Check sheet for the modelled part. Datum: model origin and axes. Units: mm. Face numbers are marked on the shaded views. A direction names the side the tool comes from. Give positions to 0.01 mm unless a question says otherwise; leave off trailing zeros. Order: outer loops, then holes, each group sorted by start corner. A loop starts at its lowest first (then second) coordinate and runs counter-clockwise, first axis right, second up.
Item 1: Sectioned sample at D-D on z = 61. Record the boundary of the cut face in (x, y).
Item 2: Access from +Z, -Z, +X, -X, +Y, -Y to the whole of each face (thin tool, end or side, straight path). Record for the marked faces 4, 5 and 6.
Item 3: Sectioned sample at A-A on y = 26. Record the boundary of the cut face in (x, z), and give its area (3 significant figures).
Item 4: Sectioned sample at C-C on y = 3. Record the boundary of the cut face in (x, z), and give its area (3 significant figures).
Item 5: Release check for a two-part mould opening along X. For the marked faces 1, 2 and 3 record: released by +X, released by -X, zero draft, split by the parting line, or undercut.
Item 6: Material ranges on line 1 along Y through (x, z) = (18, 24); line 2 along Z through (x, y) = (12.5, -4.5), recorded low to high.
Item 7: Gauge pin test, flat ends, axial feed: P1, Ø10.5, axis at x = -6, y = 8, coming from the -Z side; P2, Ø6, axis at x = -19.5, y = 17.5, coming from the -Z side; P3, Ø1.2, axis at x = 29.5, y = -3, coming from the +Z side. Record the tip position at first contact, or that the pin passes through.
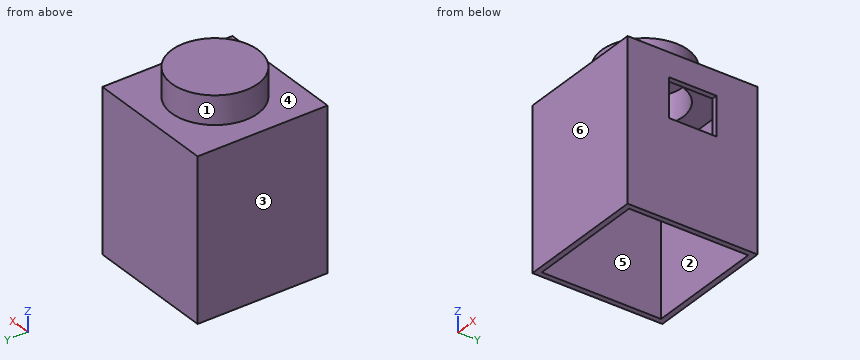
from build123d import *

# Parameters (mm, degrees)
F3_W     = 60
F3_H     = 60
F4_DEPTH = 73.86
F5_R     = 19.95
F6_DEPTH = 13.08
F8_T     = -2.5
F7_W     = 22
F7_H     = 18
F9_DEPTH = 2.5


with BuildPart() as f4:
    # F3 (on Top) → F4 (new body)
    with BuildSketch(Plane.XY):
        Rectangle(F3_W, F3_H)
    extrude(amount=F4_DEPTH)

    # F5 (on face) → F6 (join)
    with BuildSketch(Plane.XY.offset(73.86)):
        with Locations((-0.130815577, 0.1308139617)):
            Circle(F5_R)
    extrude(amount=F6_DEPTH)

    # F8
    f8_openings = [f4.faces().sort_by_distance(p)[0] for p in [
        (0, 0, 0),
    ]]
    offset(amount=F8_T, openings=f8_openings, kind=Kind.INTERSECTION)

    # F7 (on face) → F9 (cut)
    with BuildSketch(Plane.YZ.offset(30)):
        with Locations((0, 53.86)):
            Rectangle(F7_W, F7_H)
    extrude(amount=-F9_DEPTH, mode=Mode.SUBTRACT)


solid = f4.part
Report:
1. outline: (-30, -30) - (30, -30) - (30, -11) - (27.5, -11) - (27.5, -27.5) - (-27.5, -27.5) - (-27.5, 27.5) - (27.5, 27.5) - (27.5, 11) - (30, 11) - (30, 30) - (-30, 30) - close
2. face 4: +Z
2. face 5: -Z
2. face 6: +Z, -Z, +X, -X, -Y
3. outline: (-30, 0) - (-27.5, 0) - (-27.5, 71.36) - (27.5, 71.36) - (27.5, 0) - (30, 0) - (30, 73.86) - (-30, 73.86) - close
3. area: 507 mm2
4. outline: (-30, 0) - (-27.5, 0) - (-27.5, 71.36) - (-17.34, 71.36) - (-17.34, 84.44) - (17.08, 84.44) - (17.08, 71.36) - (27.5, 71.36) - (27.5, 62.86) - (30, 62.86) - (30, 73.86) - (19.61, 73.86) - (19.61, 86.94) - (-19.87, 86.94) - (-19.87, 73.86) - (-30, 73.86) - close; (27.5, 0) - (30, 0) - (30, 44.86) - (27.5, 44.86) - close
4. area: 528 mm2
5. face 1: split by the parting line
5. face 2: undercut
5. face 3: released by -X
6. line 1: y = -30 to -27.5, 27.5 to 30
6. line 2: z = 84.44 to 86.94
7. P1: stops at z = 84.44
7. P2: stops at z = 71.36
7. P3: stops at z = 73.86
